The model under review builds one solid part; all positions refer to its coordinate system, in mm. A direction names the side the tool comes from. Round coordinates to 2 decimals unless told otherwise and drop trailing zeros. Write each loop counter-clockwise with the first axis right and the second up, starting at its lowest first coordinate (ties: lowest second). Pieces come first, ordered by that corner, then holes. Notation, with made-up numbers: M 7,-26 L 14,-26 A22 ccw 14,-20 Z; hole C 83,37 d2. An arc over 180 degrees is marked long. Write item = value, one per line. Start each with the question number.
Item 1: The part is to be moulded in two halves that separate along X. For faces 3 (the cylindrical face through (0, -29, 37)), 4 (the conical face through (12.209, -23.474, 16.627)), 5 (the flat face through (19, 21, 42)), say which applies: +X half, -X half, draft (parallel to the pull), parting line (faces both ways), or undercut.
Item 2: To check wall thickness, follow line 1 along X through (y, z) = (0, 3); line 2 along Y through (x, z) = (11.5, 32.5); line 3 along Z through (x, y) = (7, 14.5). State the ranges of each line that lie inside material, in increasing order.
Item 3: Take a section at A-A, the plane y = 0. Give the boundary of the cut face in (x, z).
Item 4: Take a section at C-C, the plane z = 15. Give the boundary of the cut face in (x, y).
Item 5: Tool access review of faces 1 (the flat face through (-21, 19, 42)), 2 (the flat face through (8.2, 8.2, 12)): name each direction out of +Z, -Z, +X, -X, +Y, -Y from which nothing blocks a thin tool from reaching the whole face with its end or side.
Item 6: Take a section at D-D, the plane z = 10. Give the boundary of the cut face in (x, y), plus the area to 3 significant figures.
Item 7: For pin 1 Ø5 at (x, z) = (23.5, 29.5) entering from -Y; pin 2 Ø12 at (y, z) = (-13, 27.5) entering from -X; pin 3 Ø10 at (x, z) = (-25, 23.5) entering from +Y, all flat-tipped, find the tip position at first contact; note any pin that passes through.
Solid Edge part; units mm, degrees
sketch "Sketch1" plane through (0, 0, 0) normal (0, -1, 0) x (1, 0, 0)
  line L0 (11.25, 0) -> (22.5, 0)
  line L1 (22.5, 0) -> (32.5, 42)
  line L2 (32.5, 42) -> (26.5, 42)
  line L3 (26.5, 42) -> (19, 12)
  line L4 (19, 12) -> (11.25, 12)
  line L5 (11.25, 12) -> (11.25, 0)
  dimension "D1" = 11.25
revolve "RevolvedProtrusion1" add sketch "Sketch1" angle 360 about axis through (0, 0, 54) along (0, 0, -1)
sketch "Sketch2" plane through (0, 0, 0) normal (0, -1, 0) x (1, 0, 0)
  circle A0 centre (0, 42) radius 5
extrude "Cutout1" cut sketch "Sketch2" along normal mid plane 139.2818
sketch "Sketch3" plane through (0, 0, 0) normal (1, 0, 0) x (0, 1, 0)
  circle A0 centre (0, 42) radius 5
extrude "ExtrudedCutout_2" cut sketch "Sketch3" along normal mid plane 121.6254
properties part number "4" material "CAST STEEL"
Response values:
q1.face_3 = undercut
q1.face_4 = parting line
q1.face_5 = draft
q2.line_1 = -23.21 to -11.25, 11.25 to 23.21
q2.line_2 = -27.97 to -21.21, 21.21 to 27.97
q2.line_3 = 0 to 12
q3.outline = M -31.31,37 L -22.5,0 L -11.25,0 L -11.25,12 L -19,12 L -25.25,37 Z; M 11.25,0 L 22.5,0 L 31.31,37 L 25.25,37 L 19,12 L 11.25,12 Z
q4.outline = C 0,0 d52.14; hole C 0,0 d39.5
q5.face_1 = +Z, +X, -X, +Y, -Y
q5.face_2 = +Z
q6.outline = C 0,0 d49.76; hole C 0,0 d22.5
q6.area = 1,550 mm2
q7.pin_1 = -20.89
q7.pin_2 = -28.76
q7.pin_3 = 20.01
